from build123d import *

# Parameters (mm, degrees)
F0_W     = 75.76968
F0_H     = 25.4
F1_DEPTH = 25.4
F3_DEPTH = 31.75
F4_W     = 5.986491
F4_H     = 5.698793
F4_W_2   = 6.224596
F4_H_2   = 6.43815
F4_W_3   = 5.22054
F4_H_3   = 5.975276
F4_W_4   = 5.337961
F4_H_4   = 6.926889
F5_DEPTH = 12.7


with BuildPart() as f1:
    # F0 (on Front) → F1 (new body)
    with BuildSketch(Plane.XZ):
        Rectangle(F0_W, F0_H)
    extrude(amount=F1_DEPTH)

    # F2 (on Right) → F3 (cut, symmetric)
    with BuildSketch(Plane.YZ):
        Polygon((-6.912117, 7.487419), (-35.072637, 7.678879), (-39.277993, -27.769957), (-7.134533, -25.226125), align=None)
    extrude(amount=F3_DEPTH, both=True, mode=Mode.SUBTRACT)

    # F4 (on Front) → F5 (join)
    with BuildSketch(Plane.XZ):
        with Locations((-34.387763, 9.403795)):
            Rectangle(F4_W, F4_H)
        with Locations((-34.247685, -9.749556)):
            Rectangle(F4_W_2, F4_H_2)
        with Locations((34.564514, -9.146943)):
            Rectangle(F4_W_3, F4_H_3)
        with Locations((34.584024, 8.600718)):
            Rectangle(F4_W_4, F4_H_4)
    extrude(amount=-F5_DEPTH)


solid = f1.part
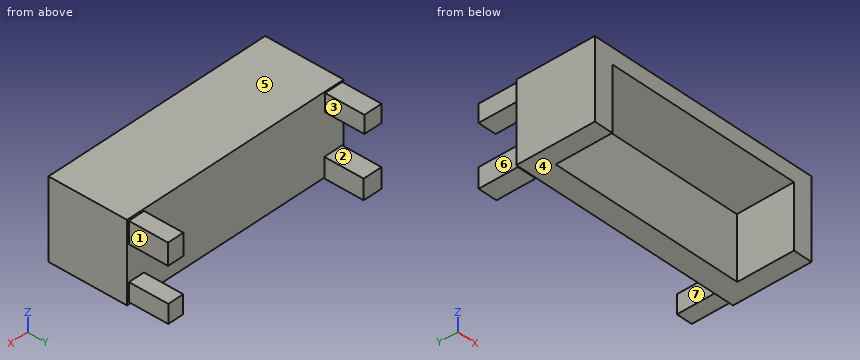
Verification items for the finished model (mm, model axes). Face numbers are marked on the shaded views. A direction names the side the tool comes from. Coordinates: 2 decimals unless noted, no trailing zeros. Order: outer loops, then holes, each group sorted by start corner. A loop starts at its lowest first (then second) coordinate and runs counter-clockwise, first axis right, second up.
1. Scan lines: line 1 (X direction, y = 2.5, z = 11.75); line 2 (X direction, y = -9.5, z = 4); line 3 (Z direction, x = 32, y = -7). Record each from-to range of solid material in increasing order.
Results found:
line 1: x = -37.38 to -31.39, 31.92 to 37.25
line 2: x = -37.88 to -31.75, 31.75 to 37.88
line 3: z = -12.7 to 12.7
2. Sectioned sample at A-A, the plane y = 4.5. Record the cut outline in (x, z), and give its area (3 significant figures).
Results found:
outline: (-37.38, 6.55) - (-31.39, 6.55) - (-31.39, 12.25) - (-37.38, 12.25) - close; (-37.36, -12.97) - (-31.14, -12.97) - (-31.14, -6.53) - (-37.36, -6.53) - close; (31.92, 5.14) - (37.25, 5.14) - (37.25, 12.06) - (31.92, 12.06) - close; (31.95, -12.13) - (37.17, -12.13) - (37.17, -6.16) - (31.95, -6.16) - close
area: 142 mm2
3. Set-up check for the marked faces 1, 2, 3 and 4: record each of +Z, -Z, +X, -X, +Y, -Y from which the full face is reachable in a straight line by a thin tool's end or side.
Results found:
face 1: +Z, -Z, +X, +Y
face 2: -X, +Y
face 3: +Z, +Y
face 4: -Z, +X, -X, -Y
4. Sectioned sample at D-D, the plane y = -13.5. Record the cut outline in (x, z).
Results found:
outline: (-37.88, -12.7) - (-31.75, -12.7) - (-31.75, 7.53) - (31.75, 7.53) - (31.75, -12.7) - (37.88, -12.7) - (37.88, 12.7) - (-37.88, 12.7) - close
5. Release check for a two-part mould opening along X. For the marked faces 5, 6 and 7 record: +X half, -X half, draft (parallel to the pull), parting line (faces both ways), or undercut.
Results found:
face 5: draft
face 6: -X half
face 7: undercut
6. Sectioned sample at B-B, the plane z = 9.25. Record the cut outline in (x, y).
Results found:
outline: (-37.88, -25.4) - (37.88, -25.4) - (37.88, 0) - (37.25, 0) - (37.25, 12.7) - (31.92, 12.7) - (31.92, 0) - (-31.39, 0) - (-31.39, 12.7) - (-37.38, 12.7) - (-37.38, 0) - (-37.88, 0) - close
7. Go/stop test with flat-tipped pins: pin 1 Ø1.6 at (x, y) = (35.5, 5.5) entering from +Z; pin 2 Ø1.7 at (y, z) = (8.5, 9.5) entering from +X; pin 3 Ø1.9 at (x, y) = (-34.5, 9.5) entering from +Z. Record where each tip stops, or that it passes through.
Results found:
pin 1: stops at z = 12.06
pin 2: stops at x = 37.25
pin 3: stops at z = 12.25
8. Sectioned sample at C-C, the plane x = 19. Record the cut outline in (y, z), and give its area (3 significant figures).
Results found:
outline: (-25.4, 7.61) - (-6.91, 7.49) - (-7.05, -12.7) - (0, -12.7) - (0, 12.7) - (-25.4, 12.7) - close
area: 272 mm2
